The listing builds one solid part. Answer for the finished solid, in the listing's coordinates (mm). Face numbers are marked on the shaded views. Round coordinates to 2 decimals unless told otherwise and drop trailing zeros. Order: outer loops, then holes, each group sorted by start corner. A loop starts at its lowest first (then second) coordinate and runs counter-clockwise, first axis right, second up. Notation, with made-up numbers: (48.5, 4) - (77.5, 4) arc R26 cw to (77.5, 41) - close; hole circle Ø9 at (72, 62). An arc over 180 degrees is marked (long way). Use CSV: the item, a comma, the result in double quotes. Start each with the question number.
Item 1: Find section A-A, the plane z = 2.4. Give the vertices of the cut face in (x, y), plus the area to 3 significant figures.
Item 2: Straight lines are drawn through the part: line 1 along Y through (x, z) = (0, 2.45); line 2 along Y through (x, z) = (-2, 1.9); line 3 along X through (y, z) = (-23, 0.9). For each, find the intervals that lie inside material, in ascending order. Write a range as [from, to].
Item 3: Find section D-D, the plane y = 25. Give the vertices of the cut face in (x, z), plus the area to 3 significant figures.
Item 4: Determine the mould class of the marked faces 1, 2 and 3 for opening direction Y: +Y half, -Y half, draft (parallel to the pull), parting line (faces both ways), or undercut.
Item 5: Flat-ended cylindrical pins translate along their axes: P1, Ø1, axis at x = -2, z = 4, coming from the +Y side; P2, Ø1, axis at x = -10, z = 1.5, coming from the -Y side; P3, Ø1, axis at x = 5.5, z = 4, coming from the +Y side; P4, Ø10, axis at x = 3, y = 17.5, coming from the -Z side. Find the tip coordinate at first contact, or state that the pin passes through.
Item 6: Find section C-C, the plane y = -22. Give the vertices of the cut face in (x, z), plus the area to 3 significant figures.
Item 7: Find section B-B, the plane x = 0. Give the vertices of the cut face in (y, z), plus the area to 3 significant figures.
```python
from build123d import *

# Parameters (mm, degrees)
SKETCH1_R           = 4
BOSS_EXTRUDE1_DEPTH = 5


with BuildPart() as part:
    # Sketch1 → Boss-Extrude1 (new body)
    # profile 1 of 11: a face of its own
    with BuildSketch(Plane.XY):
        with BuildLine():
            ThreePointArc((7, 25), (-1.657831686, 18.199147546), (-6.214741171, 28.221333912))
            Line((-6.214741171, 28.221333912), (-15.878201673, 9.578154573))
            ThreePointArc((-15.878201673, 9.578154573), (-16.715503506, 7.344579965), (-17, 4.976248984))
            Line((-17, 4.976248984), (-17, -4.976248984))
            ThreePointArc((-17, -4.976248984), (-16.715503506, -7.344579965), (-15.878201673, -9.578154573))
            Line((-15.878201673, -9.578154573), (-6.214741171, -28.221333912))
            ThreePointArc((-6.214741171, -28.221333912), (-1.657831686, -18.199147546), (7, -25))
            ThreePointArc((7, -25), (6.97123748, -25.633914815), (6.885186288, -26.262620205))
            Line((6.885186288, -26.262620205), (8.835980411, -15.624757058))
            ThreePointArc((8.835980411, -15.624757058), (8.958910686, -14.7266065), (9, -13.821013908))
            Line((9, -13.821013908), (9, 13.821013908))
            ThreePointArc((9, 13.821013908), (8.958910686, 14.7266065), (8.835980411, 15.624757058))
            Line((8.835980411, 15.624757058), (6.885186288, 26.262620205))
            ThreePointArc((6.885186288, 26.262620205), (6.97123748, 25.633914815), (7, 25))
        make_face()
    # profile 2 of 11: a face of its own
    with BuildSketch(Plane.XY):
        with BuildLine():
            ThreePointArc((6.885186288, 26.262620205), (1.035139609, 31.923040227), (-6.214741171, 28.221333912))
            ThreePointArc((-6.214741171, 28.221333912), (-1.657831686, 18.199147546), (7, 25))
            ThreePointArc((7, 25), (6.97123748, 25.633914815), (6.885186288, 26.262620205))
        make_face()
        with Locations((0, 25)):
            Circle(SKETCH1_R, mode=Mode.SUBTRACT)
    # profile 3 of 11: a face of its own
    with BuildSketch(Plane.XY):
        with BuildLine():
            ThreePointArc((6.885186288, 26.262620205), (1.035139609, 31.923040227), (-6.214741171, 28.221333912))
            ThreePointArc((-6.214741171, 28.221333912), (-1.657831686, 18.199147546), (7, 25))
            ThreePointArc((7, 25), (6.97123748, 25.633914815), (6.885186288, 26.262620205))
        make_face()
        with Locations((0, 25)):
            Circle(SKETCH1_R, mode=Mode.SUBTRACT)
    # profile 4 of 11: a face of its own
    with BuildSketch(Plane.XY):
        with BuildLine():
            ThreePointArc((6.885186288, 26.262620205), (1.035139609, 31.923040227), (-6.214741171, 28.221333912))
            ThreePointArc((-6.214741171, 28.221333912), (-1.657831686, 18.199147546), (7, 25))
            ThreePointArc((7, 25), (6.97123748, 25.633914815), (6.885186288, 26.262620205))
        make_face()
        with Locations((0, 25)):
            Circle(SKETCH1_R, mode=Mode.SUBTRACT)
    # profile 5 of 11: a face of its own
    with BuildSketch(Plane.XY):
        with BuildLine():
            ThreePointArc((6.885186288, 26.262620205), (1.035139609, 31.923040227), (-6.214741171, 28.221333912))
            ThreePointArc((-6.214741171, 28.221333912), (-1.657831686, 18.199147546), (7, 25))
            ThreePointArc((7, 25), (6.97123748, 25.633914815), (6.885186288, 26.262620205))
        make_face()
        with Locations((0, 25)):
            Circle(SKETCH1_R, mode=Mode.SUBTRACT)
    # profile 6 of 11: a face of its own
    with BuildSketch(Plane.XY):
        with BuildLine():
            ThreePointArc((6.885186288, 26.262620205), (1.035139609, 31.923040227), (-6.214741171, 28.221333912))
            ThreePointArc((-6.214741171, 28.221333912), (-1.657831686, 18.199147546), (7, 25))
            ThreePointArc((7, 25), (6.97123748, 25.633914815), (6.885186288, 26.262620205))
        make_face()
        with Locations((0, 25)):
            Circle(SKETCH1_R, mode=Mode.SUBTRACT)
    # profile 7 of 11: a face of its own
    with BuildSketch(Plane.XY):
        with BuildLine():
            ThreePointArc((7, -25), (-1.657831686, -18.199147546), (-6.214741171, -28.221333912))
            ThreePointArc((-6.214741171, -28.221333912), (1.035139609, -31.923040227), (6.885186288, -26.262620205))
            ThreePointArc((6.885186288, -26.262620205), (6.97123748, -25.633914815), (7, -25))
        make_face()
        with Locations((0, -25)):
            Circle(SKETCH1_R, mode=Mode.SUBTRACT)
    # profile 8 of 11: a face of its own
    with BuildSketch(Plane.XY):
        with BuildLine():
            ThreePointArc((7, -25), (-1.657831686, -18.199147546), (-6.214741171, -28.221333912))
            ThreePointArc((-6.214741171, -28.221333912), (1.035139609, -31.923040227), (6.885186288, -26.262620205))
            ThreePointArc((6.885186288, -26.262620205), (6.97123748, -25.633914815), (7, -25))
        make_face()
        with Locations((0, -25)):
            Circle(SKETCH1_R, mode=Mode.SUBTRACT)
    # profile 9 of 11: a face of its own
    with BuildSketch(Plane.XY):
        with BuildLine():
            ThreePointArc((7, -25), (-1.657831686, -18.199147546), (-6.214741171, -28.221333912))
            ThreePointArc((-6.214741171, -28.221333912), (1.035139609, -31.923040227), (6.885186288, -26.262620205))
            ThreePointArc((6.885186288, -26.262620205), (6.97123748, -25.633914815), (7, -25))
        make_face()
        with Locations((0, -25)):
            Circle(SKETCH1_R, mode=Mode.SUBTRACT)
    # profile 10 of 11: a face of its own
    with BuildSketch(Plane.XY):
        with BuildLine():
            ThreePointArc((7, -25), (-1.657831686, -18.199147546), (-6.214741171, -28.221333912))
            ThreePointArc((-6.214741171, -28.221333912), (1.035139609, -31.923040227), (6.885186288, -26.262620205))
            ThreePointArc((6.885186288, -26.262620205), (6.97123748, -25.633914815), (7, -25))
        make_face()
        with Locations((0, -25)):
            Circle(SKETCH1_R, mode=Mode.SUBTRACT)
    # profile 11 of 11: a face of its own
    with BuildSketch(Plane.XY):
        with BuildLine():
            ThreePointArc((7, -25), (-1.657831686, -18.199147546), (-6.214741171, -28.221333912))
            ThreePointArc((-6.214741171, -28.221333912), (1.035139609, -31.923040227), (6.885186288, -26.262620205))
            ThreePointArc((6.885186288, -26.262620205), (6.97123748, -25.633914815), (7, -25))
        make_face()
        with Locations((0, -25)):
            Circle(SKETCH1_R, mode=Mode.SUBTRACT)
    extrude(amount=BOSS_EXTRUDE1_DEPTH)


solid = part.part
```
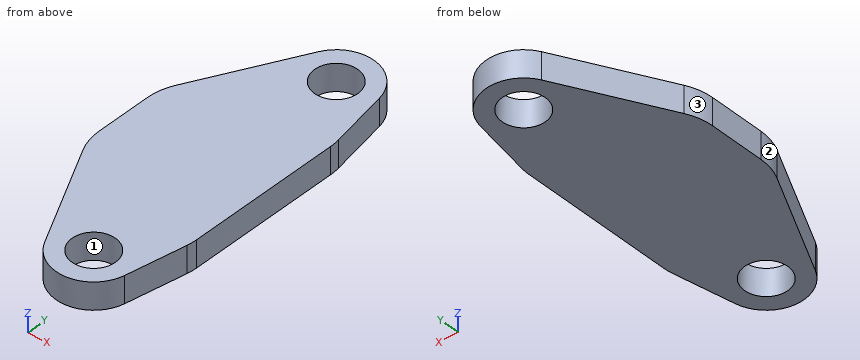
Worked out:
1,outline,"(-17, -4.98) arc R10 ccw to (-15.88, -9.58) - (-6.21, -28.22) arc R7 ccw to (6.89, -26.26) - (8.84, -15.62) arc R10 ccw to (9, -13.82) - (9, 13.82) arc R10 ccw to (8.84, 15.62) - (6.89, 26.26) arc R7 ccw to (-6.21, 28.22) - (-15.88, 9.58) arc R10 ccw to (-17, 4.98) - close; hole circle Ø8 at (0, -25); hole circle Ø8 at (0, 25)"
1,area,"1,170 mm²"
2,line 1,"y = [-32, -29], [-21, 21], [29, 32]"
2,line 2,"y = [-31.71, -28.46], [-21.54, 21.54], [28.46, 31.71]"
2,line 3,"x = [-8.92, -3.46], [3.46, 7.48]"
3,outline,"(-7.88, 0) - (-4, 0) - (-4, 5) - (-7.88, 5) - close; (4, 0) - (7.12, 0) - (7.12, 5) - (4, 5) - close"
3,area,"35.0 mm²"
4,face 1,"undercut"
4,face 2,"-Y half"
4,face 3,"+Y half"
5,P1,"stops at y = 31.84"
5,P2,"stops at y = -21.88"
5,P3,"stops at y = 29.9"
5,P4,"stops at z = 0"
6,outline,"(-9.44, 0) - (-2.65, 0) - (-2.65, 5) - (-9.44, 5) - close; (2.65, 0) - (7.67, 0) - (7.67, 5) - (2.65, 5) - close"
6,area,"59.1 mm²"
7,outline,"(-32, 0) - (-29, 0) - (-29, 5) - (-32, 5) - close; (-21, 0) - (21, 0) - (21, 5) - (-21, 5) - close; (29, 0) - (32, 0) - (32, 5) - (29, 5) - close"
7,area,"240 mm²"
